Here's how the part is built. I have some questions about the finished solid (model axes, mm). A direction names the side the tool comes from. Coordinates: 2 decimals unless noted, no trailing zeros. Write each loop counter-clockwise with the first axis right and the second up, starting at its lowest first coordinate (ties: lowest second). Pieces come first, ordered by that corner, then holes. Notation, with made-up numbers: M -14,-5.5 L 29,-5.5 A11 cw 29,15.5 Z; hole C 12.5,87 d8. An arc over 180 degrees is marked long. Use one line per item in the form item = value. Start each with the question number.
1. I'm going to push flat-ended pins straight in: pin 1 Ø3 at (x, z) = (-0.74, -13.79) entering from +Y; pin 2 Ø0.9 at (y, z) = (24.5, 11.5) entering from -X; pin 3 Ø2.5 at (y, z) = (24, 19.5) entering from +X. Where does each tip first touch, or does it pass through?
2. I want a section at A-A, the plane y = 15. List the corners of the cut face in (x, z) for me, plus the area to 3 significant figures.
3. I want a section at B-B, the plane x = 11. List the corners of the cut face in (y, z) for me.
4. Thinking about a two-plate mould opening in Z: for faces 4 (the face through (70.252, 24.192, -44.861)), 5 (the face through (31.265, 48.516, -43.277)), 6 (the face through (6.8, 22.1, -23.7)), which applies, released by +Z, released by -Z, zero draft, split by the parting line, or undercut?
5. I want a section at C-C, the plane z = 30. List the corners of the cut face in (x, y) for me, plus the area to 3 significant figures.
6. Please list where these lines run through material, in increasing order: line 1 along Z through (x, y) = (51.5, 14); line 2 along Y through (x, z) = (40, 58); line 3 along X through (y, z) = (16, 21). Write a range as [from, to].
7. On a 3-axis mill with a long thin cutter (end or side, diameter ignored), from which of +Z, -Z, +X, -X, +Y, -Y can I reach the whole of each face in a straight line? I mean faces 1 (the face through (31.27, 21.74, -24.03)), 2 (the face through (-0.66, 21.52, 54.19)), 3 (the face through (32.245, 1.504, 62.287)). Say none if no direction works.
from build123d import *

# Parameters (mm, degrees)
SKETCH_1_W          = 80
SKETCH_1_H          = 110
EXTRUDE_1_DEPTH     = 26
EXTRUDE_2_DEPTH     = 80
FILLET_1_R          = 5
SKETCH_4_W          = 70
SKETCH_4_H          = 100
CUT_EXTRUDE_1_DEPTH = 20
CUT_EXTRUDE_START   = -3.244680851
CUT_EXTRUDE_2_DEPTH = 70
SKETCH_8_W          = 60
SKETCH_8_H          = 65
CUT_EXTRUDE_3_DEPTH = 20
SKETCH_9_W          = 70
SKETCH_9_H          = 8.485281375
EXTRUDE_3_DEPTH     = 5
SKETCH_11_W         = 70
SKETCH_11_H         = 5
EXTRUDE_4_DEPTH     = 5
SKETCH_13_W         = 70
SKETCH_13_H         = 75
CUT_EXTRUDE_4_DEPTH = 3
SKETCH_14_W         = 70
SKETCH_14_H         = 30.355339059
CUT_EXTRUDE_5_DEPTH = 3
SKETCH_15_W         = 70
SKETCH_15_H         = 3
EXTRUDE_5_DEPTH     = 100
SKETCH_16_R         = 2.025
CUT_EXTRUDE_6_DEPTH = 5
SKETCH_17_R         = 2.025
CUT_EXTRUDE_7_DEPTH = 5
SKETCH_18_R         = 2.25
CUT_EXTRUDE_8_DEPTH = 45


# Read off the part's stored shape, not the designer's step: the extrude step
with BuildPart() as part:
    # Sketch 1 → Extrude 1 (new body)
    with BuildSketch(Plane(origin=(0, 0, 0), x_dir=(1, 0, 0), z_dir=(0, 1, 0))):
        with Locations((31.755319149, -8.712765957)):
            Rectangle(SKETCH_1_W, SKETCH_1_H)
    extrude(amount=EXTRUDE_1_DEPTH)

    # Sketch 2 → Extrude 2 (add)
    with BuildSketch(Plane(origin=(71.755319149, 0, 0), x_dir=(0, 0, -1), z_dir=(1, 0, 0))):
        Polygon((46.287234043, 26), (46.287234043, 56), (16.287234043, 26), align=None)
    extrude(amount=-EXTRUDE_2_DEPTH)

    # Fillet 1
    fillet_1_edges = [part.edges().sort_by_distance(p)[0] for p in [
        (71.755319149, 26, 23.712765957),
        (-8.244680851, 26, 23.712765957),
        (-8.244680851, 41, -31.287234043),
        (31.755319149, 56, -46.287234043),
        (71.755319149, 41, -31.287234043),
        (31.755319149, 0, -46.287234043),
        (71.755319149, 0, 8.712765957),
        (31.755319149, 0, 63.712765957),
        (-8.244680851, 0, 8.712765957),
        (-8.244680851, 28, -46.287234043),
        (71.755319149, 28, -46.287234043),
        (71.755319149, 13, 63.712765957),
        (-8.244680851, 13, 63.712765957),
        (31.755319149, 26, 63.712765957),
    ]]
    fillet(fillet_1_edges, radius=FILLET_1_R)

    # Sketch 4 → Cut-Extrude 1 (cut)
    with BuildSketch(Plane.XZ):
        with Locations((31.755319149, 8.712765957)):
            Rectangle(SKETCH_4_W, SKETCH_4_H)
    extrude(amount=-CUT_EXTRUDE_1_DEPTH, mode=Mode.SUBTRACT)

    # Cut-Extrude 2 outline → Cut-Extrude 2 (cut)
    with BuildSketch(Plane.YZ.offset(CUT_EXTRUDE_START)):
        Polygon((20, -22.287234043), (20, -41.287234043), (43.928932188, -41.287234043), (47.464466094, -37.751700137), (26, -16.287234043), align=None)
    extrude(amount=CUT_EXTRUDE_2_DEPTH, mode=Mode.SUBTRACT)

    # Sketch 8 → Cut-Extrude 3 (cut)
    with BuildSketch(Plane(origin=(0, 26, 0), x_dir=(1, 0, 0), z_dir=(0, 1, 0))):
        with Locations((31.755319149, -21.212765957)):
            Rectangle(SKETCH_8_W, SKETCH_8_H)
    extrude(amount=-CUT_EXTRUDE_3_DEPTH, mode=Mode.SUBTRACT)

    # Sketch 9 → Extrude 3 (add)
    with BuildSketch(Plane(origin=(0, 21.143617021, -21.143617021), x_dir=(1, 0, 0), z_dir=(0, 0.7071067811865511, -0.707106781186544))):
        with Locations((31.755319149, -2.625321985)):
            Rectangle(SKETCH_9_W, SKETCH_9_H)
    extrude(amount=EXTRUDE_3_DEPTH)

    # Sketch 11 → Extrude 4 (add)
    with BuildSketch(Plane(origin=(0, 42.608083115, -42.608083115), x_dir=(1, 0, 0), z_dir=(0, -0.7071067811865511, 0.707106781186544))):
        with Locations((31.755319149, 4.367962673)):
            Rectangle(SKETCH_11_W, SKETCH_11_H)
    extrude(amount=EXTRUDE_4_DEPTH)

    # Sketch 13 → Cut-Extrude 4 (cut)
    with BuildSketch(Plane(origin=(0, 26, 0), x_dir=(1, 0, 0), z_dir=(0, 1, 0))):
        with Locations((31.755319149, -21.212765957)):
            Rectangle(SKETCH_13_W, SKETCH_13_H)
    extrude(amount=-CUT_EXTRUDE_4_DEPTH, mode=Mode.SUBTRACT)

    # Sketch 14 → Cut-Extrude 5 (cut)
    with BuildSketch(Plane(origin=(0, 4.856382979, 4.856382979), x_dir=(1, 0, 0), z_dir=(0, 0.7071067811865441, 0.7071067811865509))):
        with Locations((31.755319149, 45.079259479)):
            Rectangle(SKETCH_14_W, SKETCH_14_H)
    extrude(amount=-CUT_EXTRUDE_5_DEPTH, mode=Mode.SUBTRACT)

    # Sketch 15 → Extrude 5 (add)
    with BuildSketch(Plane.XY.offset(-41.287234043)):
        with Locations((31.755319149, 1.5)):
            Rectangle(SKETCH_15_W, SKETCH_15_H)
    extrude(amount=EXTRUDE_5_DEPTH)

    # Sketch 16 → Cut-Extrude 6 (cut)
    with BuildSketch(Plane(origin=(0, 2.735062635, 2.735062635), x_dir=(1, 0, 0), z_dir=(0, 0.7071067811865444, 0.7071067811865508))):
        with Locations(Location((6.755319149, 57.756929008, 0), (0, 0, 270))):
            Circle(SKETCH_16_R)
        with Locations(Location((56.755319149, 57.756929008, 0), (0, 0, 270))):
            Circle(SKETCH_16_R)
        with Locations(Location((31.755319149, 57.756929008, 0), (0, 0, 270))):
            Circle(SKETCH_16_R)
        with Locations(Location((6.755319149, 32.401589949, 0), (0, 0, 270))):
            Circle(SKETCH_16_R)
        with Locations(Location((56.755319149, 32.401589949, 0), (0, 0, 270))):
            Circle(SKETCH_16_R)
        with Locations(Location((31.755319149, 32.401589949, 0), (0, 0, 270))):
            Circle(SKETCH_16_R)
    extrude(amount=-CUT_EXTRUDE_6_DEPTH, mode=Mode.SUBTRACT)

    # Sketch 17 → Cut-Extrude 7 (cut)
    with BuildSketch(Plane(origin=(0, 23, 0), x_dir=(1, 0, 0), z_dir=(0, 1, 0))):
        with Locations(Location((-0.744680851, 13.787234043, 0), (0, 0, 270))):
            Circle(SKETCH_17_R)
        with Locations(Location((64.255319149, -56.212765957, 0), (0, 0, 270))):
            Circle(SKETCH_17_R)
        with Locations(Location((-0.744680851, -56.212765957, 0), (0, 0, 270))):
            Circle(SKETCH_17_R)
        with Locations(Location((64.255319149, 13.787234043, 0), (0, 0, 270))):
            Circle(SKETCH_17_R)
    extrude(amount=-CUT_EXTRUDE_7_DEPTH, mode=Mode.SUBTRACT)

    # Sketch 18 → Cut-Extrude 8 (cut)
    with BuildSketch(Plane(origin=(0, 0, -46.287234043), x_dir=(-1, 0, 0), z_dir=(0, 0, -1))):
        with Locations((-31.755319149, 10.25)):
            Circle(SKETCH_18_R)
    extrude(amount=-CUT_EXTRUDE_8_DEPTH, mode=Mode.SUBTRACT)


solid = part.part
Answer list:
q1.pin_1 = 3
q1.pin_2 = -7.21
q1.pin_3 = 71.44
q2.outline = M -8.24,-41.29 A5 ccw -3.24,-46.29 L 66.76,-46.29 A5 ccw 71.76,-41.29 L 71.76,58.71 A5 ccw 66.76,63.71 L -3.24,63.71 A5 ccw -8.24,58.71 Z; hole M -3.24,-41.29 L 66.76,-41.29 L 66.76,58.71 L -3.24,58.71 Z
q2.area = 1,780 mm²
q3.outline = M 0,-41.29 A5 ccw 5,-46.29 L 43.93,-46.29 A5 ccw 47.46,-37.75 L 45.34,-39.87 L 41.81,-36.34 L 40.39,-37.75 L 43.93,-41.29 L 3,-41.29 L 3,58.71 L 20,58.71 L 20,53.71 L 23,53.71 L 23,58.71 L 26,58.71 A5 ccw 21,63.71 L 5,63.71 A5 ccw 0,58.71 Z; M 20,-22.29 L 23.54,-25.82 L 27.41,-21.94 L 23.88,-18.41 L 26,-16.29 L 23,-16.29 L 23,-11.29 L 20,-11.29 Z
q4.face_4 = released by -Z
q4.face_5 = split by the parting line
q4.face_6 = undercut
q5.outline = M -8.24,5 A5 ccw -3.24,0 L 66.76,0 A5 ccw 71.76,5 L 71.76,21 A5 ccw 66.76,26 L 66.76,23 L 61.76,23 L 61.76,20 L 66.76,20 L 66.76,3 L -3.24,3 L -3.24,20 L 1.76,20 L 1.76,23 L -3.24,23 L -3.24,26 A5 ccw -8.24,21 Z
q5.area = 479 mm²
q6.line_1 = [-46.29, -41.29], [58.71, 63.71]
q6.line_2 = [0, 3], [20, 23]
q6.line_3 = [-8.24, -3.24], [66.76, 71.76]
q7.face_1 = none
q7.face_2 = +Y
q7.face_3 = +Z, +X, -X, -Y
